from build123d import *

# Parameters (mm, degrees)
F1_DEPTH = 25
F3_DEPTH = 6
F4_R     = 3
F5_DEPTH = 6
F6_W     = 5
F6_H     = 15
F7_DEPTH = 13
F8_R     = 2.5
F9_DEPTH = 25


with BuildPart() as f1:
    # F0 (on Right) → F1 (new body)
    with BuildSketch(Plane.YZ):
        with BuildLine():
            Line((0, 6), (0, 0))
            Line((0, 0), (40, 0))
            Line((40, 0), (40, 31))
            Line((40, 31), (34, 31))
            Line((34, 31), (34, 8.5))
            ThreePointArc((34, 8.5), (33.267767, 6.732233), (31.5, 6))
            Line((31.5, 6), (0, 6))
        make_face()
    extrude(amount=F1_DEPTH)

    # F2 (on face) → F3 (cut)
    with BuildSketch(Plane(origin=(0, 40, 0), x_dir=(-1, 0, 0), z_dir=(0, 1, 0))):
        Polygon((-25, 31), (-25, 15), (-20, 31), align=None)
        with BuildLine():
            Line((-9, 21), (-9, 31))
            Line((-9, 31), (-12.5, 31))
            Line((-12.5, 31), (-16, 31))
            Line((-16, 31), (-16, 21))
            ThreePointArc((-16, 21), (-12.5, 17.5), (-9, 21))
        make_face()
        Polygon((-5, 31), (0, 15), (0, 31), align=None)
        Polygon((-9, 31), (-5, 31), (0, 31), (0, 32), (-25, 32), (-25, 31), (-20, 31), (-16, 31), (-12.5, 31), align=None)
    extrude(amount=-F3_DEPTH, mode=Mode.SUBTRACT)

    # F4 (on face) → F5 (cut)
    with BuildSketch(Plane.XY.offset(6)):
        with Locations((12.5, 25)):
            Circle(F4_R)
        with Locations((12.5, 7.5)):
            Circle(F4_R)
    extrude(amount=-F5_DEPTH, mode=Mode.SUBTRACT)

    # F6 (on face) → F7 (join)
    with BuildSketch(Plane(origin=(0, 40, 0), x_dir=(-1, 0, 0), z_dir=(0, 1, 0))):
        with Locations((-22.5, 7.5)):
            Rectangle(F6_W, F6_H)
        with Locations((-2.5, 7.5)):
            Rectangle(F6_W, F6_H)
    extrude(amount=F7_DEPTH)

    # F8 (on face) → F9 (cut)
    with BuildSketch(Plane.YZ.offset(25)):
        with BuildLine():
            ThreePointArc((48.163654, 13.386077), (51.635835, 11.309073), (53, 7.5))
            Line((53, 7.5), (53, 15))
            Line((53, 15), (40, 15))
            Line((40, 15), (48.163654, 13.386077))
        make_face()
        with Locations((47, 7.5)):
            Circle(F8_R)
        with BuildLine():
            Line((48.163654, 1.613923), (40, 0))
            Line((40, 0), (47, 0))
            Line((47, 0), (53, 0))
            Line((53, 0), (53, 7.5))
            ThreePointArc((53, 7.5), (51.635835, 3.690927), (48.163654, 1.613923))
        make_face()
    extrude(amount=-F9_DEPTH, mode=Mode.SUBTRACT)


solid = f1.part
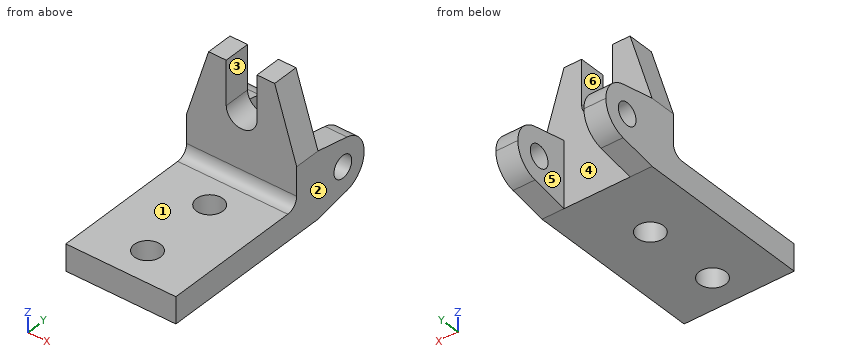
The model under review builds one solid part; all positions refer to its coordinate system, in mm. Face numbers are marked on the shaded views. A direction names the side the tool comes from. Round coordinates to 2 decimals unless told otherwise and drop trailing zeros. Loops run counter-clockwise (first coordinate to the right, second up) from the corner with the lowest first, then second, coordinate; pieces in that order, holes last. Notation, with made-up numbers: (-25.75, 16) - (-5.75, 16) arc R18 cw to (-5.75, 42) - close; hole circle Ø6 at (4, 74). An arc over 180 degrees is marked (long way). Use CSV: the item, a comma, the result in double quotes.
(1) Take a section at A-A, the plane x = 12.5. Give the boundary of the cut face in (y, z).
Working result:
outline,"(0, 0) - (4.5, 0) - (4.5, 6) - (0, 6) - close; (10.5, 0) - (22, 0) - (22, 6) - (10.5, 6) - close; (28, 0) - (40, 0) - (40, 17.5) - (34, 17.5) - (34, 8.5) arc R2.5 cw to (31.5, 6) - (28, 6) - close"
(2) Clearance check with flat-ended pins moving along their axes: P1, Ø4, axis at x = 22.5, y = 13, coming from the +Z side; P2, Ø5, axis at y = 37.5, z = 24, coming from the -X side; P3, Ø6, axis at x = 17.5, z = 9.5, coming from the -Y side. State where each tip first meets the part, or that it passes through.
Working result:
P1,"stops at z = 6"
P2,"stops at x = 2.03"
P3,"stops at y = 33"
(3) Machinability: for the marked faces 4, 5 and 6, which of the approach directions +Z, -Z, +X, -X, +Y, -Y give a long, thin tool a straight path to every point of the face, cutting with its end or side? Answer none if there is none.
Working result:
face 4,"+Z, +Y"
face 5,"+Z, -Z, +Y"
face 6,"+Z, +Y, -Y"
(4) Take a section at B-B, the plane y = 25. Give the boundary of the cut face in (x, z).
Working result:
outline,"(0, 0) - (9.5, 0) - (9.5, 6) - (0, 6) - close; (15.5, 0) - (25, 0) - (25, 6) - (15.5, 6) - close"
(5) The part is to be moulded in two halves that separate along X. For the marked faces 1, 2 and 3, say which applies: pulls with the +X half, pulls with the -X half, needs draft (parallel to the pull), parting line crosses it, or undercut.
Working result:
face 1,"needs draft"
face 2,"pulls with the +X half"
face 3,"undercut"
(6) Take a section at D-D, the plane x = 2.75. Give the boundary of the cut face in (y, z).
Working result:
outline,"(0, 0) - (40, 0) - (48.16, 1.61) arc R6 ccw to (53, 7.5) arc R6 ccw to (48.16, 13.39) - (40, 15) - (40, 23.8) - (34, 23.8) - (34, 8.5) arc R2.5 cw to (31.5, 6) - (0, 6) - close; hole circle Ø5 at (47, 7.5)"
(7) Take a section at C-C, the plane z = 27.5. Give the boundary of the cut face in (x, y), plus the area to 3 significant figures.
Working result:
outline,"(3.91, 34) - (9, 34) - (9, 40) - (3.91, 40) - close; (16, 34) - (21.09, 34) - (21.09, 40) - (16, 40) - close"
area,"61.1 mm^2"
(8) For line 1 (Y direction, x = 12.5, z = 4.25); line 2 (X direction, y = 50, z = 12); line 3 (Z direction, x = 2.25, y = 31.5), list the stretches that pass through material, from the lowest coordinate up.
Working result:
line 1,"y = 0 to 4.5, 10.5 to 22, 28 to 40"
line 2,"x = 0 to 5, 20 to 25"
line 3,"z = 0 to 6"
